CAD build for the part. Positions are in the model's coordinates, mm. Face numbers are marked on the shaded views. A direction names the side the tool comes from. Round coordinates to 2 decimals unless told otherwise and drop trailing zeros. Loops run counter-clockwise (first coordinate to the right, second up) from the corner with the lowest first, then second, coordinate; pieces in that order, holes last. Notation, with made-up numbers: M -4,-40 L 48,-40 A13 ccw 48,-19 Z; hole C 58,-3 d6. An arc over 180 degrees is marked long. Use a Markdown table: item, result. Add a question column.
(1) Band-saw the part on C-C, the plane y = 12.5. Write the cut outline in (x, z), and give its area (3 significant figures).
(2) Which spindle directions (+Z, -Z, +X, -X, +Y, -Y) get a long thin tool onto all of the face, cutting with end or side? Do the marked faces 1, 2 and 3. Say none if no direction does.
(3) Band-saw the part on D-D, the plane y = 7.25. Write the cut outline in (x, z), and give its area (3 significant figures).
(4) Flat gauge pins, fed straight in: P1, Ø5, axis at x = 9, z = 11, coming from the +Y side; P2, Ø9, axis at x = -2, y = 16, coming from the +Z side; P3, Ø5, axis at y = 13, z = -1, coming from the +X side; P4, Ø2, axis at y = 12.5, z = 2.5, coming from the -X side. Where does each tip first touch, or does it go through?
(5) Two-plate mould, pull along Y, no slides. Class the marked faces 4, 5 and 6: released by +Y, released by -Y, zero draft, split by the parting line, or undercut.
(6) Band-saw the part on A-A, the plane z = 9.5. Write the cut outline in (x, y), and give its area (3 significant figures).
(7) Band-saw the part on B-B, the plane y = 15. Write the cut outline in (x, z).
(8) Wall check: L1, parallel to X at y = 14.75, z = -7.75; L2, parallel to Z at x = -1, y = 17; L3, parallel to X at y = 13, z = -11.25. Give the ranges that are in metal, low to high.
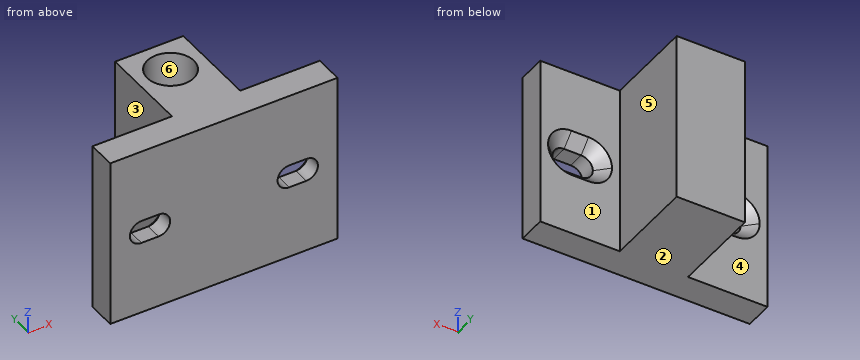
from build123d import *

# Parameters (mm, degrees)
SKIZZE1_W                                      = 40
SKIZZE1_H                                      = 30
AUFSATZ_LINEAR_AUSTRAGEN1_DEPTH                = 5
SKIZZE3_W                                      = 12
SKIZZE3_H                                      = 30
AUFSATZ_LINEAR_AUSTRAGEN2_DEPTH                = 16
SKIZZE4_R                                      = 4.1
SCHNITT_LINEAR_AUSTRAGEN1_DEPTH                = 25
FORMSENKUNG_LANGLOCH_F_R_M3_SENKSCHRAUBE_DEPTH = 5


with BuildPart() as part:
    # Skizze1 → Aufsatz-Linear austragen1 (new body)
    with BuildSketch(Plane(origin=(0, 0, 0), x_dir=(1, 0, 0), z_dir=(0, 1, 0))):
        Rectangle(SKIZZE1_W, SKIZZE1_H)
    extrude(amount=AUFSATZ_LINEAR_AUSTRAGEN1_DEPTH)

    # Skizze3 → Aufsatz-Linear austragen2 (add)
    with BuildSketch(Plane(origin=(0, 5, 0), x_dir=(1, 0, 0), z_dir=(0, 1, 0))):
        Rectangle(SKIZZE3_W, SKIZZE3_H)
    extrude(amount=AUFSATZ_LINEAR_AUSTRAGEN2_DEPTH)

    # Skizze4 → Schnitt-Linear austragen1 (cut)
    with BuildSketch(Plane.XY.offset(15)):
        with Locations((0, 15)):
            Circle(SKIZZE4_R)
    extrude(amount=-SCHNITT_LINEAR_AUSTRAGEN1_DEPTH, mode=Mode.SUBTRACT)

    # Formsenkung Langloch für M3 Senkschraube mit Schlitz/Kreuzschlitz1: read off the stored shape, not the designer's step
    # Formsenkung Langloch f_r M3 Senkschr 2 → Formsenkung Langloch für M3 Senkschraube mit Schlitz/Kreuzschlitz1 (cut)
    with BuildSketch(Plane(origin=(0, 0, 0), x_dir=(1, 0, 0), z_dir=(0, 1, 0))):
        with BuildLine():
            Line((-14.5, -2.05), (-11.5, -2.05))
            ThreePointArc((-11.5, -2.05), (-9.45, 0), (-11.5, 2.05))
            Line((-11.5, 2.05), (-14.5, 2.05))
            ThreePointArc((-14.5, 2.05), (-16.55, 0), (-14.5, -2.05))
        make_face()
    formsenkung_langloch_f_r_m3_senkschraube = extrude(amount=FORMSENKUNG_LANGLOCH_F_R_M3_SENKSCHRAUBE_DEPTH, mode=Mode.SUBTRACT)

    # Formsenkung Langloch f_r M3 Senkschr 3: loft between two sections, ruled curve by curve
    formsenkung_langloch_f_r_m3_senkschr_3_from = [
        Edge.make_three_point_arc((-11.5, 2.925, 2.05), (-10.050431099, 2.925, 1.449568901), (-9.45, 2.925, 0)),
        Edge.make_three_point_arc((-9.45, 2.925, 0), (-10.050431099, 2.925, -1.449568901), (-11.5, 2.925, -2.05)),
        Edge.make_three_point_arc((-14.5, 2.925, -2.05), (-15.949568901, 2.925, -1.449568901), (-16.55, 2.925, 0)),
        Edge.make_three_point_arc((-16.55, 2.925, 0), (-15.949568901, 2.925, 1.449568901), (-14.5, 2.925, 2.05)),
        Edge.make_line((-11.5, 2.925, -2.05), (-14.5, 2.925, -2.05)),
        Edge.make_line((-11.5, 2.925, 2.05), (-14.5, 2.925, 2.05)),
    ]
    formsenkung_langloch_f_r_m3_senkschr_3_to = [
        Edge.make_three_point_arc((-11.5, 5, 4.125), (-8.583184528, 5, 2.916815472), (-7.375, 5, 0)),
        Edge.make_three_point_arc((-7.375, 5, 0), (-8.583184528, 5, -2.916815472), (-11.5, 5, -4.125)),
        Edge.make_three_point_arc((-14.5, 5, -4.125), (-17.416815472, 5, -2.916815472), (-18.625, 5, 0)),
        Edge.make_three_point_arc((-18.625, 5, 0), (-17.416815472, 5, 2.916815472), (-14.5, 5, 4.125)),
        Edge.make_line((-11.5, 5, -4.125), (-14.5, 5, -4.125)),
        Edge.make_line((-11.5, 5, 4.125), (-14.5, 5, 4.125)),
    ]
    formsenkung_langloch_f_r_m3_senkschr_3 = Solid(Shell([*[Face.make_surface_from_curves(formsenkung_langloch_f_r_m3_senkschr_3_from[k], formsenkung_langloch_f_r_m3_senkschr_3_to[k]) for k in range(6)], Face(Wire(formsenkung_langloch_f_r_m3_senkschr_3_from)), Face(Wire(formsenkung_langloch_f_r_m3_senkschr_3_to))]))
    add(formsenkung_langloch_f_r_m3_senkschr_3, mode=Mode.SUBTRACT)

    # Spiegeln1: Formsenkung Langloch für M3 Senkschraube mit Schlitz/Kreuzschlitz1, Formsenkung Langloch f_r M3 Senkschr 3 across plane
    add(formsenkung_langloch_f_r_m3_senkschraube.mirror(Plane(origin=(0, 0, 0), x_dir=(0, 0, 1), z_dir=(1, 0, 0))), mode=Mode.SUBTRACT)
    add(formsenkung_langloch_f_r_m3_senkschr_3.mirror(Plane(origin=(0, 0, 0), x_dir=(0, 0, 1), z_dir=(1, 0, 0))), mode=Mode.SUBTRACT)


solid = part.part
Return value:
| question | item | result |
|---|---|---|
| 1 | outline | M -6,-15 L 6,-15 L 6,15 L 3.25,15 L 3.25,-10 L -3.25,-10 L -3.25,15 L -6,15 Z |
| 1 | area | 198 mm^2 |
| 2 | face 1 | +Z, -Z, +X, +Y |
| 2 | face 2 | -Z, +X, -X, +Y, -Y |
| 2 | face 3 | +Z, -Z, -X, +Y |
| 3 | outline | M -6,-15 L 6,-15 L 6,15 L -6,15 Z |
| 3 | area | 360 mm^2 |
| 4 | P1 | y = 5 |
| 4 | P2 | z = 15 |
| 4 | P3 | x = 6 |
| 4 | P4 | x = -6 |
| 5 | face 4 | released by +Y |
| 5 | face 5 | zero draft |
| 5 | face 6 | undercut |
| 6 | outline | M -20,0 L 20,0 L 20,5 L 6,5 L 6,21 L -6,21 L -6,5 L -20,5 Z; hole C 0,15 d8.2 |
| 6 | area | 339 mm^2 |
| 7 | outline | M -6,-15 L 6,-15 L 6,15 L 4.1,15 L 4.1,-10 L -4.1,-10 L -4.1,15 L -6,15 Z |
| 8 | L1 | -6 to -4.09, 4.09 to 6 |
| 8 | L2 | -15 to -10 |
| 8 | L3 | -6 to 6 |
